from build123d import *

# Parameters (mm, degrees)
SKETCH1_W               = 15
SKETCH1_H               = 10
SKETCH1_R               = 1.5
BOSS_EXTRUDE1_DEPTH     = 5
SKETCH2_R               = 1.5
CUT_EXTRUDE1_DEPTH      = 1
CUT_EXTRUDE1_DEPTH_BACK = 16
SKETCH3_R               = 1.5
CUT_EXTRUDE2_DEPTH      = 1
CUT_EXTRUDE2_DEPTH_BACK = 11
SKETCH4_W               = 10
SKETCH4_H               = 5
CUT_EXTRUDE3_DEPTH      = 4.75


with BuildPart() as part:
    # Sketch1 → Boss-Extrude1 (new body)
    with BuildSketch(Plane(origin=(0, 0, 0), x_dir=(1, 0, 0), z_dir=(0, 1, 0))):
        Rectangle(SKETCH1_W, SKETCH1_H)
        with Locations((4, 0)):
            Circle(SKETCH1_R, mode=Mode.SUBTRACT)
        with Locations((-4, 0)):
            Circle(SKETCH1_R, mode=Mode.SUBTRACT)
    extrude(amount=BOSS_EXTRUDE1_DEPTH)

    # Sketch2 → Cut-Extrude1 (cut, two sides)
    with BuildSketch(Plane.ZY.offset(7.5)) as cut_extrude1_sk:
        with Locations((0, 2.5)):
            Circle(SKETCH2_R)
    extrude(amount=CUT_EXTRUDE1_DEPTH, mode=Mode.SUBTRACT)
    extrude(cut_extrude1_sk.sketch, amount=-CUT_EXTRUDE1_DEPTH_BACK, mode=Mode.SUBTRACT)

    # Sketch3 → Cut-Extrude2 (cut, two sides)
    with BuildSketch(Plane(origin=(0, 0, -5), x_dir=(-1, 0, 0), z_dir=(0, 0, -1))) as cut_extrude2_sk:
        with Locations((0, 2.5)):
            Circle(SKETCH3_R)
    extrude(amount=CUT_EXTRUDE2_DEPTH, mode=Mode.SUBTRACT)
    extrude(cut_extrude2_sk.sketch, amount=-CUT_EXTRUDE2_DEPTH_BACK, mode=Mode.SUBTRACT)

    # Sketch4 → Cut-Extrude3 (cut)
    with BuildSketch(Plane.ZY.offset(7.5)):
        with Locations((0, 2.5)):
            Rectangle(SKETCH4_W, SKETCH4_H)
    extrude(amount=-CUT_EXTRUDE3_DEPTH, mode=Mode.SUBTRACT)


solid = part.part
Work out the finished part from the listing and answer in its coordinate system (mm). Give positions to 0.01 mm unless a question says otherwise; leave off trailing zeros. Loops run counter-clockwise (first coordinate to the right, second up) from the corner with the lowest first, then second, coordinate; pieces in that order, holes last. Notation, with made-up numbers: (-5.5, 89) -> (39.5, 89) arc R24 ccw to (39.5, 101) -> close; hole circle Ø9 at (36, 38). An arc over 180 degrees is marked (long way). Use a Markdown table: item, result. Add a question column.
1. Section D-D on y = 0.8 is taken. Determine the outline of the cut face in (x, z).
2. Find the intervals of material crossed by probe 1 along Y at (x, z) = (2, 0); probe 2 along Z at (x, y) = (4, 1.95); probe 3 along X at (y, z) = (2.5, 3.5), in increasing order.
3. Section C-C on y = 3.2 is taken. Determine the outline of the cut face in (x, z).
4. Determine the mould class of faces 1 (the flat face through (2, 2, 5)), 2 (the cylindrical face through (3.675, 0.955, 1.464)), 3 (the flat face through (7.5, 1, 1)), 4 (the flat face through (-2.75, 3, -3)) for opening direction X: released by +X, released by -X, zero draft, split by the parting line, or undercut.
5. Section B-B on x = -2 is taken. Determine the outline of the cut face in (y, z).
6. Section A-A on z = -2.25 is taken. Determine the outline of the cut face in (x, y), and give its area (3 significant figures).
7. A flat-ended cylindrical pin translates along its axis: pin 1 Ø1.8 at (y, z) = (2.5, 0) entering from -X. Find the tip coordinate at first contact, or state that the pin passes through.
Results below:
| question | item | result |
|---|---|---|
| 1 | outline | (-2.75, -5) -> (7.5, -5) -> (7.5, 5) -> (-2.75, 5) -> (-2.75, 0.83) arc R1.5 cw to (-2.75, -0.83) -> close; hole circle Ø3 at (4, 0) |
| 2 | probe 1 | y = 0 to 1, 4 to 5 |
| 2 | probe 2 | z = -5 to -1.5, 1.5 to 5 |
| 2 | probe 3 | x = -2.75 to -1.5, 1.5 to 7.5 |
| 3 | outline | (-2.75, -5) -> (-1.33, -5) -> (-1.33, -1.33) -> (-2.75, -1.33) -> close; (-2.75, 1.33) -> (-1.33, 1.33) -> (-1.33, 5) -> (-2.75, 5) -> close; (1.33, -5) -> (7.5, -5) -> (7.5, -1.33) -> (4.7, -1.33) arc R1.5 cw to (3.3, -1.33) -> (1.33, -1.33) -> close; (1.33, 1.33) -> (3.3, 1.33) arc R1.5 cw to (4.7, 1.33) -> (7.5, 1.33) -> (7.5, 5) -> (1.33, 5) -> close |
| 4 | face 1 | zero draft |
| 4 | face 2 | undercut |
| 4 | face 3 | released by +X |
| 4 | face 4 | released by -X |
| 5 | outline | (0, -5) -> (5, -5) -> (5, 5) -> (0, 5) -> close; hole circle Ø3 at (2.5, 0) |
| 6 | outline | (-2.75, 0) -> (7.5, 0) -> (7.5, 5) -> (-2.75, 5) -> close; hole circle Ø3 at (0, 2.5) |
| 6 | area | 44.2 mm^2 |
| 7 | pin 1 | passes through |
